from build123d import *

# Parameters (mm, degrees)
CHAMFER_1_SIZE      = 1
SKETCH_2_W          = 13.14097419
SKETCH_2_H          = 3.873114836
CUT_EXTRUDE_1_DEPTH = 6.5


with BuildPart() as part:
    # 草图1 → 旋转1 (revolve)
    with BuildSketch(Plane.XY, mode=Mode.PRIVATE) as revolve_1_sk:
        with BuildLine():
            Line((4.131730263, 5.65055794), (5, 8.175))
            Line((5, 8.175), (5, 12.175))
            Line((5, 12.175), (3, 12.175))
            Line((3, 12.175), (3, 18.175))
            Line((3, 18.175), (2, 18.175))
            Line((2, 18.175), (2, 19.175))
            Line((2, 19.175), (3, 19.175))
            Line((3, 19.175), (3, 30.175))
            Line((3, 30.175), (0, 30.175))
            Line((0, 30.175), (0, -7))
            ThreePointArc((0, -7), (6.654092935, -2.173257281), (4.131730263, 5.65055794))
        make_face()
    revolve(revolve_1_sk.sketch.rotate(Axis((0, 30.175, 0), (0, -1, 0)), 90), axis=Axis((0, 30.175, 0), (0, -1, 0)))

    # 倒角1
    chamfer_1_edges = [part.edges().sort_by_distance(p)[0] for p in [
        (0, 30.175, -3),
    ]]
    chamfer(chamfer_1_edges, length=CHAMFER_1_SIZE)

    # 草图2 → 切除-拉伸1 (cut)
    with BuildSketch(Plane(origin=(0, 12.175, 0), x_dir=(1, 0, 0), z_dir=(0, 1, 0))):
        with Locations((1.143581663, -5.936557418)):
            Rectangle(SKETCH_2_W, SKETCH_2_H)
        with Locations((1.143581663, 5.936557418)):
            Rectangle(SKETCH_2_W, SKETCH_2_H)
    extrude(amount=-CUT_EXTRUDE_1_DEPTH, mode=Mode.SUBTRACT)


solid = part.part
Verification items for the finished model (mm, model axes). A direction names the side the tool comes from. Coordinates: 2 decimals unless noted, no trailing zeros. Loops run counter-clockwise (first coordinate to the right, second up) from the corner with the lowest first, then second, coordinate; pieces in that order, holes last. Notation, with made-up numbers: (-11, 75.5) -> (38, 75.5) arc R30 ccw to (38, 111.5) -> close; hole circle Ø10 at (-21, 26.5). An arc over 180 degrees is marked (long way). Answer as CSV lines item,"result".
1) Depth check by flat-ended pin: pin 1 (5 mm diameter, centred on x = -2, z = -2.5, fed in from -Y); pin 2 (4 mm diameter, centred on x = -2.5, z = 3.5, fed in from +Y); pin 3 (6 mm diameter, centred on y = 9.5, z = -5.5, fed in from -X). Enter the tip coordinate at first touch or a pass-through.
Found:
pin 1,"stops at y = -6.96"
pin 2,"stops at y = 29.87"
pin 3,"stops at x = -4.33"
2) Release check for a two-part mould opening along Y. For faces 1 (the flat face through (-3.4, 12.175, -0.1)), 2 (the conical face through (2.55, 5.81, -3.32)), 3 (the flat face through (0, 9, 4)), 4 (the flat face through (2, 19.175, -1)) record: +Y half, -Y half, draft (parallel to the pull), parting line (faces both ways), or undercut.
Found:
face 1,"+Y half"
face 2,"undercut"
face 3,"draft"
face 4,"undercut"
3) Cross-section at D-D, the plane y = 11. Record the cut outline in (x, z), then the cut area to 3 significant figures.
Found:
outline,"(-3, -4) -> (3, -4) arc R5 ccw to (3, 4) -> (-3, 4) arc R5 ccw to start"
area,"70.4 mm2"
4) Cross-section at A-A, the plane z = 0. Record the cut outline in (x, y) (3 decimals).
Found:
outline,"(-5, 8.175) -> (-4.132, 5.651) arc R7 ccw (long way) to (4.132, 5.651) -> (5, 8.175) -> (5, 12.175) -> (3, 12.175) -> (3, 18.175) -> (2, 18.175) -> (2, 19.175) -> (3, 19.175) -> (3, 29.175) -> (2, 30.175) -> (-2, 30.175) -> (-3, 29.175) -> (-3, 19.175) -> (-2, 19.175) -> (-2, 18.175) -> (-3, 18.175) -> (-3, 12.175) -> (-5, 12.175) -> close"
5) Thickness scan on L1, parallel to Y at x = 2.5, z = 3.5 (3 decimals); L2, parallel to Y at x = 6, z = 2; L3, parallel to Z at x = -2.25, y = 9.5. Record the ranges inside material, lowest first. Write a range as from..to.
Found:
L1,"y = -5.523..5.523, 6.143..12.175"
L2,"y = -3..3"
L3,"z = -4..4"
6) Cross-section at C-C, the plane y = 25. Record the cut outline in (x, z).
Found:
outline,"circle Ø6 at (0, 0)"
7) Tool access check on faces 5 (the cylindrical face through (-5, 10, 0)), 6 (the cylindrical face through (5, 10, 0)), 7 (the cylindrical face through (2, 19, 0)), 8 (the cylindrical face through (-0.9, 24.24, 2.86)). Record the directions out of +Z, -Z, +X, -X, +Y, -Y that give a thin tool (end or side, any length) a straight path to the whole face; none if there is none.
Found:
face 5,"-X, +Y"
face 6,"+X, +Y"
face 7,"none"
face 8,"+Y"
8) Cross-section at B-B, the plane x = 0. Record the cut outline in (y, z) (3 decimals).
Found:
outline,"(5.651, -4.132) -> (5.675, -4.14) -> (5.675, -4) -> (12.175, -4) -> (12.175, -3) -> (18.175, -3) -> (18.175, -2) -> (19.175, -2) -> (19.175, -3) -> (29.175, -3) -> (30.175, -2) -> (30.175, 2) -> (29.175, 3) -> (19.175, 3) -> (19.175, 2) -> (18.175, 2) -> (18.175, 3) -> (12.175, 3) -> (12.175, 4) -> (5.675, 4) -> (5.675, 4.14) -> (5.651, 4.132) arc R7 ccw (long way) to start"
